Autodesk Inventor part; units mm, degrees
ref_plane "YZ Plane" through (0, 0, 0) normal (1, 0, 0) x (0, 1, 0)
ref_plane "XZ Plane" through (0, 0, 0) normal (0, 1, 0) x (-1, 0, 0)
ref_plane "XY Plane" through (0, 0, 0) normal (0, 0, 1) x (1, 0, 0)
sketch "Sketch1" plane through (0, 0, 0) normal (0, 1, 0) x (-1, 0, 0)
  line L0 (25, 25) -> (-25, 25)
  line L1 (-25, 25) -> (-25, -25)
  line L2 (-25, -25) -> (25, -25)
  line L3 (25, -25) -> (25, 25)
  point P0 (0, 0)
  dimension "d0" = 25
  dimension "d1" = 50
  dimension "d2" = 25
  dimension "d3" = 25
extrude "Extrusion1" add sketch "Sketch1" along normal blind 50
sketch "Sketch2" plane through (0, 50, 0) normal (0, 1, 0) x (1, 0, 0)
  line L0 (-22, -22) -> (22, -22)
  line L1 (22, -22) -> (22, 22)
  line L2 (22, 22) -> (-22, 22)
  line L3 (-22, 22) -> (-22, -22)
  point P0 (0, 0)
  dimension "d6" = 22
  dimension "d7" = 22
  dimension "d8" = 22
  dimension "d9" = 22
extrude "Extrusion2" cut sketch "Sketch2" against normal blind 47
sketch "Sketch3" plane through (0, 3, 0) normal (0, 1, 0) x (1, 0, 0)
  circle A0 centre (0, 0) radius 5
  dimension "d12" = 10
extrude "Extrusion3" add sketch "Sketch3" along normal blind 40
sketch "Sketch4" plane through (0, 50, 0) normal (0, 1, 0) x (1, 0, 0)
  line L0 (-22, 22) -> (22, 22)
  line L1 (22, 22) -> (22, 25)
  line L2 (22, 25) -> (-22, 25)
  line L3 (-22, 25) -> (-22, 22)
  line L4 (25, -25) -> (25, 25)
  point P0 (0, 0)
  dimension "d15" = 3
  dimension "d16" = 25
extrude "Extrusion4" cut sketch "Sketch4" against normal blind 3
sketch "Sketch5" plane through (-22, 3, -22) normal (0, 0, 1) x (1, 0, 0)
  point P0 (22, -3)
sketch "Sketch6" plane through (25, 0, -25) normal (0, 0, -1) x (-1, 0, 0)
  line L0 (3, 47) -> (47, 47)
  circle A0 centre (25, 47) radius 2
  point P0 (25, 0)
  dimension "d19" = 4
extrude "Extrusion5" cut sketch "Sketch6" against normal blind 3
sketch "Sketch7" plane through (-22, 50, 22) normal (1, 0, 0) x (0, 0, -1)
  point P0 (22, -50)
sketch "Sketch8" plane through (25, 0, -25) normal (0, 0, -1) x (-1, 0, 0)
  line L0 (47, 50) -> (47, 47)
  circle A0 centre (47, 48.5) radius 0.75
  line L1 (3, 50) -> (47, 50)
  line L2 (3, 47) -> (3, 50)
  circle A1 centre (3, 48.5) radius 0.75
  point P0 (25, 0)
  dimension "d22" = 1.5
  dimension "d23" = 1.5
  dimension "d24" = 1.5
extrude "Extrusion6" cut sketch "Sketch8" against normal blind 48.5 contours A0 L0 | L0 A0
sketch "Sketch9" plane through (25, 0, -25) normal (0, 0, -1) x (-1, 0, 0)
  point P0 (25, 0)
sketch "Sketch10" plane through (25, 0, -25) normal (0, 0, -1) x (-1, 0, 0)
  line L0 (3, 50) -> (3, 3)
  circle A0 centre (3, 48.5) radius 0.75
  line L1 (3, 50) -> (47, 50)
  point P0 (25, 0)
  dimension "d27" = 1.5
  dimension "d28" = 1.5
extrude "Extrusion7" cut sketch "Sketch10" against normal blind 48.5
sketch "Sketch11" plane through (22, 50, 22) normal (0, 0, -1) x (-1, 0, 0)
  line L0 (44, -0.75) -> (0, -0.75)
  line L1 (0, -0.75) -> (0, -2.25)
  line L2 (0, -2.25) -> (44, -2.25)
  line L3 (44, -2.25) -> (44, -0.75)
  point P0 (22, -50)
extrude "Extrusion8" cut sketch "Sketch11" against normal blind 1.5
sketch "Sketch12" plane through (0, 3, 0) normal (0, 1, 0) x (1, 0, 0)
  line L0 (-21.9343, 35.7574) -> (18.5832, 35.7574)
  line L1 (18.5832, 35.7574) -> (18.5832, 64.5461)
  line L2 (18.5832, 64.5461) -> (-21.9343, 64.5461)
  line L3 (-21.9343, 64.5461) -> (-21.9343, 35.7574)
  point P0 (0, 0)
properties part number "Box01"
Source: CAD feature listing. Evaluate the final solid. Frame: model axes, mm. A direction names the side the tool comes from. Give positions to 0.01 mm unless a question says otherwise; leave off trailing zeros. Write each loop counter-clockwise with the first axis right and the second up, starting at its lowest first coordinate (ties: lowest second). Pieces come first, ordered by that corner, then holes.
1. Section query D-D (z = -10). Return the cut outline in (x, y), then the cut area to 3 significant figures.
2. Pull-direction query (X, two-part tool) for faces 1 (the face through (0, 26, 22)), 2 (the face through (25, 25, 0)), 3 (the face through (0, 25, -25)); classes: +X half, -X half, draft (parallel to the pull), parting line (faces both ways), or undercut.
3. Access query for faces 4 (the face through (0, 25, -22)), 5 (the face through (0, 45, -24)), 6 (the face through (-25, 25, 0)), 7 (the face through (0, 0, 0)), 8 (the face through (0, 49, 23.5)). Directions: +Z, -Z, +X, -X, +Y, -Y. A direction counts if a zero-diameter tool reaches every point of the face in a straight line with its end or side. Return the directions, or none.
4. Material intervals for line 1 along Z through (x, y) = (-9.5, 8); line 2 along Z through (x, y) = (3, 27), sorted ascending.
5. Section query A-A (y = 40). Return the cut outline in (x, z), then the cut area to 3 significant figures.
6. Section query C-C (x = 0). Return the cut outline in (y, z).
7. Section query B-B (z = 0). Return the cut outline in (x, y), then the cut area to 3 significant figures.
8. First-contact query: pin 1 (3.5 mm diameter, centred on x = -14.5, z = -24, fed in from +Y); pin 2 (8 mm diameter, centred on x = 17.5, z = -5.5, fed in from +Y); pin 3 (13 mm diameter, centred on x = 7, z = 4.5, fed in from +Y). Flat tips, straight axial feed; report the tip coordinate or a pass-through.
Output values:
1. outline: (-25, 0) - (25, 0) - (25, 50) - (22, 50) - (22, 49.25) arc R0.75 cw to (22, 47.75) - (22, 3) - (-22, 3) - (-22, 47.75) arc R0.75 cw to (-22, 49.25) - (-22, 50) - (-25, 50) - close
1. area: 430 mm2
2. face 1: undercut
2. face 2: +X half
2. face 3: draft
3. face 4: +Y
3. face 5: -Z, +Y
3. face 6: +Z, -Z, -X, +Y, -Y
3. face 7: +Z, -Z, +X, -X, -Y
3. face 8: -Z
4. line 1: z = -25 to -22, 22 to 25
4. line 2: z = -25 to -22, -4 to 4, 22 to 25
5. outline: (-25, -25) - (25, -25) - (25, 25) - (-25, 25) - close; circle Ø10 at (0, 0); hole (-22, -22) - (22, -22) - (22, 22) - (-22, 22) - close
5. area: 643 mm2
6. outline: (0, -25) - (45, -25) - (45, -22) - (3, -22) - (3, -5) - (43, -5) - (43, 5) - (3, 5) - (3, 22) - (47.75, 22) - (47.75, 23.5) - (49.25, 23.5) - (49.25, 22) - (50, 22) - (50, 25) - (0, 25) - close
7. outline: (-25, 0) - (25, 0) - (25, 50) - (22, 50) - (22, 49.25) arc R0.75 cw to (22, 47.75) - (22, 3) - (5, 3) - (5, 43) - (-5, 43) - (-5, 3) - (-22, 3) - (-22, 47.75) arc R0.75 cw to (-22, 49.25) - (-22, 50) - (-25, 50) - close
7. area: 830 mm2
8. pin 1: stops at y = 47
8. pin 2: stops at y = 3
8. pin 3: stops at y = 43
